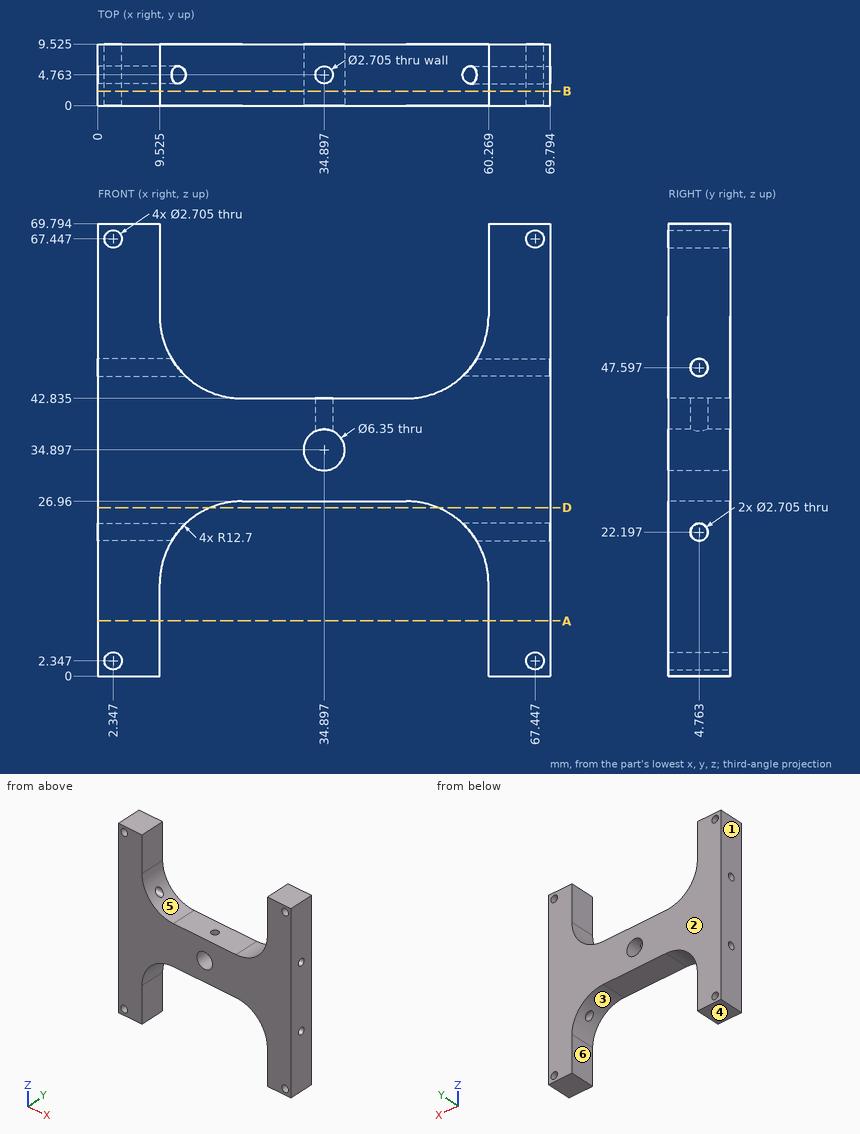
Geometry: see drawing. Coordinates: mm, zero at the bounding-box minimum. A direction names the side the tool comes from. Give positions to 0.01 mm unless a question says otherwise; leave off trailing zeros. Order: outer loops, then holes, each group sorted by start corner. A loop starts at its lowest first (then second) coordinate and runs counter-clockwise, first axis right, second up. Notation, with made-up numbers: M 65,-18.5 L 80,-18.5 A21 cw 80,-0.5 Z; hole C -5,13 d10. An arc over 180 degrees is marked long. Answer as CSV lines item,"result". Start each with the question number.
1) Cut plane B-B (y = 2.25). State how many separate pieces and enclosed holes the cut face has, then the cut area to 3 significant figures.
2) Set-up query: the marked faces 4, 5 and 6. Return all of +Z, -Z, +X, -X, +Y, -Y with unobstructed straight access to the full face (end or side cutting, diameter ignored); none if empty.
3) First-contact query: P1, Ø5, axis at x = 38.5, y = 3.5, coming from the +Z side (1 decimal); P2, Ø4, axis at x = 12, z = 16.5, coming from the +Y side; P3, Ø1.5, axis at x = 58.5, y = 6, coming from the -Z side (1 decimal); P4, Ø3, axis at x = 34.9, y = 4.76, coming from the -Z side. Flat tips, straight axial feed; report the tip coordinate or a pass-through.
4) Cut plane D-D (z = 26). Output: boundary loops of the cut face in (x, y) (1 decimal), then the cut area to 3 significant figures.
5) Mould query, pull axis X, two halves, no side actions, for the marked faces 1, 2 and 3. Classes: +X half, -X half, draft (parallel to the pull), parting line (faces both ways), or undercut.
6) Line query: line 1 (X direction, y = 5, z = 7) (1 decimal); line 2 (X direction, y = 2.25, z = 67) (1 decimal); line 3 (Z direction, x = 36, y = 7.75) (1 decimal). Output: solid intervals per line, ascending. Write a range as from..to.
7) Cut plane A-A (z = 8.5). Output: boundary loops of the cut face in (x, y) (1 decimal).
Findings below:
1,separate pieces,"1"
1,enclosed holes,"5"
1,area,"2,220 mm²"
2,face 4,"-Z, +X, -X, +Y, -Y"
2,face 5,"+Z, +Y, -Y"
2,face 6,"-Z, +Y, -Y"
3,P1,"stops at z = 42.8"
3,P2,"passes through"
3,P3,"stops at z = 19.2"
3,P4,"stops at z = 26.96"
4,outline,"M 0,0 L 17.4,0 L 17.4,9.5 L 0,9.5 Z; M 52.4,0 L 69.8,0 L 69.8,9.5 L 52.4,9.5 Z"
4,area,"331 mm²"
5,face 1,"-X half"
5,face 2,"draft"
5,face 3,"undercut"
6,line 1,"x = 0..9.5, 60.3..69.8"
6,line 2,"x = 0..1.1, 3.6..9.5, 60.3..66.2, 68.7..69.8"
6,line 3,"z = 27..31.9, 37.9..42.8"
7,outline,"M 0,0 L 9.5,0 L 9.5,9.5 L 0,9.5 Z; M 60.3,0 L 69.8,0 L 69.8,9.5 L 60.3,9.5 Z"
